Input: part model. Units: mm. Frame: model coordinates. A direction names the side the tool comes from. Coordinates: 2 decimals unless noted, no trailing zeros. Order: outer loops, then holes, each group sorted by start corner. A loop starts at its lowest first (then second) coordinate and runs counter-clockwise, first axis right, second up.
from build123d import *

# Parameters (mm, degrees)
SKETCH1_W                      = 76
SKETCH1_H                      = 32
BOSS_EXTRUDE1_DEPTH            = 13
SKETCH2_R                      = 6
CUT_EXTRUDE1_DEPTH             = 1
CUT_EXTRUDE1_DEPTH_BACK        = 14
SKETCH3_W                      = 82
SKETCH3_H                      = 39
BOSS_EXTRUDE2_DEPTH            = 13
SKETCH4_W                      = 82
SKETCH4_H                      = 13
BOSS_EXTRUDE3_DEPTH            = 87
SKETCH5_W                      = 68
SKETCH5_H                      = 50
CUT_EXTRUDE2_DEPTH             = 1
CUT_EXTRUDE2_DEPTH_BACK        = 40
SKETCH6_W                      = 13
SKETCH6_H                      = 32
BOSS_EXTRUDE4_DEPTH            = 41
FILLET1_R                      = 6
CUT_EXTRUDE3_REACH             = 178
CUT_EXTRUDE3_DIRECTION_2_DEPTH = 1


with BuildPart() as part:
    # Sketch1 → Boss-Extrude1 (new body)
    with BuildSketch(Plane(origin=(0, 0, 0), x_dir=(1, 0, 0), z_dir=(0, 1, 0))):
        Rectangle(SKETCH1_W, SKETCH1_H)
    extrude(amount=BOSS_EXTRUDE1_DEPTH)

    # Sketch2 → Cut-Extrude1 (cut, two sides)
    with BuildSketch(Plane(origin=(0, 13, 0), x_dir=(1, 0, 0), z_dir=(0, 1, 0))) as cut_extrude1_sk:
        with Locations((-22, 0)):
            Circle(SKETCH2_R)
        with Locations((22, 0)):
            Circle(SKETCH2_R)
    extrude(amount=CUT_EXTRUDE1_DEPTH, mode=Mode.SUBTRACT)
    extrude(cut_extrude1_sk.sketch, amount=-CUT_EXTRUDE1_DEPTH_BACK, mode=Mode.SUBTRACT)

    # Sketch3 → Boss-Extrude2 (add)
    with BuildSketch(Plane.ZY.offset(38)):
        with Locations((25, 19.5)):
            Rectangle(SKETCH3_W, SKETCH3_H)
    extrude(amount=BOSS_EXTRUDE2_DEPTH)

    # Sketch4 → Boss-Extrude3 (add)
    with BuildSketch(Plane.ZY.offset(51)):
        with Locations((25, 32.5)):
            Rectangle(SKETCH4_W, SKETCH4_H)
    extrude(amount=BOSS_EXTRUDE3_DEPTH)

    # Sketch5 → Cut-Extrude2 (cut, two sides)
    with BuildSketch(Plane(origin=(0, 39, 0), x_dir=(1, 0, 0), z_dir=(0, 1, 0))) as cut_extrude2_sk:
        with Locations((-104, -9)):
            Rectangle(SKETCH5_W, SKETCH5_H)
    extrude(amount=CUT_EXTRUDE2_DEPTH, mode=Mode.SUBTRACT)
    extrude(cut_extrude2_sk.sketch, amount=-CUT_EXTRUDE2_DEPTH_BACK, mode=Mode.SUBTRACT)

    # Sketch6 → Boss-Extrude4 (add)
    with BuildSketch(Plane.XZ.offset(-26)):
        with Locations((-131.5, 50)):
            Rectangle(SKETCH6_W, SKETCH6_H)
    extrude(amount=BOSS_EXTRUDE4_DEPTH)

    # Fillet1
    fillet1_edges = [part.edges().sort_by_distance(p)[0] for p in [
        (-51, 26, 25),
        (-38, 6.5, 16),
        (-125, 26, 50),
    ]]
    fillet(fillet1_edges, radius=FILLET1_R)

    # Sketch7 → Cut-Extrude3 (cut, up to next)
    with BuildSketch(Plane.ZY.offset(138), mode=Mode.PRIVATE) as cut_extrude3_sk1:
        with BuildLine():
            Line((43, 0), (43, -15))
            Line((43, -15), (57, -15))
            Line((57, -15), (57, 0))
            ThreePointArc((57, 0), (50, 7), (43, 0))
        make_face()
    cut_extrude3_tool1 = extrude(cut_extrude3_sk1.sketch, amount=-CUT_EXTRUDE3_REACH, mode=Mode.PRIVATE) & part.part
    add(cut_extrude3_tool1.solids().sort_by_distance((-138, -4.691563, 50))[0], mode=Mode.SUBTRACT)

    # Sketch7 → Cut-Extrude3 direction 2 (cut)
    with BuildSketch(Plane.ZY.offset(138)):
        with BuildLine():
            Line((43, 0), (43, -15))
            Line((43, -15), (57, -15))
            Line((57, -15), (57, 0))
            ThreePointArc((57, 0), (50, 7), (43, 0))
        make_face()
    extrude(amount=CUT_EXTRUDE3_DIRECTION_2_DEPTH, mode=Mode.SUBTRACT)


solid = part.part
Item 1: Draft query along Z for faces 4 (the face through (38, 6, 0)), 5 (the face through (-15, 11, -16)), 6 (the face through (17.24, 6.59, 3.65)). Return one class per face: pulls with the +Z half, pulls with the -Z half, needs draft (parallel to the pull), parting line crosses it, or undercut.
Response values:
face 4: needs draft
face 5: pulls with the -Z half
face 6: undercut
Item 2: Cut plane C-C on x = 22. Return loops of the section in (y, z).
Response values:
outline: (0, -16) - (13, -16) - (13, -6) - (0, -6) - close; (0, 6) - (13, 6) - (13, 16) - (0, 16) - close
Item 3: Access query for faces 1 (the face through (-132, -7, 43)), 2 (the face through (-120, 30, 34)), 3 (the face through (-51, 10, 24)). Directions: +Z, -Z, +X, -X, +Y, -Y. A direction counts if a zero-diameter tool reaches every point of the face in a straight line with its end or side. Return the directions, or none.
Response values:
face 1: +X, -X, -Y
face 2: -Z, -X, +Y, -Y
face 3: +Z, -Z, -Y
Item 4: Pin query (flat end, axial travel): pin 1 Ø10.5 at (x, y) = (-133.5, -9.5) entering from -Z; pin 2 Ø8 at (y, z) = (28, 10.5) entering from -X; pin 3 Ø19 at (x, z) = (-5.5, -1.5) entering from +Y; pin 4 Ø4 at (y, z) = (-3, 47.5) entering from +X. Return the tip coordinate at first contact, or that it passes through.
Response values:
pin 1: stops at z = 34
pin 2: stops at x = -70
pin 3: stops at y = 13
pin 4: passes through
Item 5: Cut plane D-D on z = -8.5. Return loops of the section in (x, y).
Response values:
outline: (-70, 26) - (-57, 26) arc R6 cw to (-51, 20) - (-51, 0) - (38, 0) - (38, 13) - (-38, 13) - (-38, 39) - (-70, 39) - close
Item 6: Cut plane B-B on z = 0. Return loops of the section in (x, y).
Response values:
outline: (-70, 26) - (-57, 26) arc R6 cw to (-51, 20) - (-51, 0) - (-28, 0) - (-28, 13) - (-38, 13) - (-38, 39) - (-70, 39) - close; (-16, 0) - (16, 0) - (16, 13) - (-16, 13) - close; (28, 0) - (38, 0) - (38, 13) - (28, 13) - close
Item 7: Cut plane A-A on y = -5. Return loops of the section in (x, z), then the cut area to 3 significant figures.
Response values:
outline: (-138, 34) - (-125, 34) - (-125, 43) - (-138, 43) - close; (-138, 57) - (-125, 57) - (-125, 66) - (-138, 66) - close
area: 234 mm2
Item 8: Ray query, probe 1 along X at (y, z) = (7.5, 0); probe 2 along Z at (x, y) = (22, 5.25); probe 3 along X at (y, z) = (-1.5, 40.5). Return the intervals inside material, ascending.
Response values:
probe 1: x = -51 to -28, -16 to 16, 28 to 38
probe 2: z = -16 to -6, 6 to 16
probe 3: x = -138 to -125
